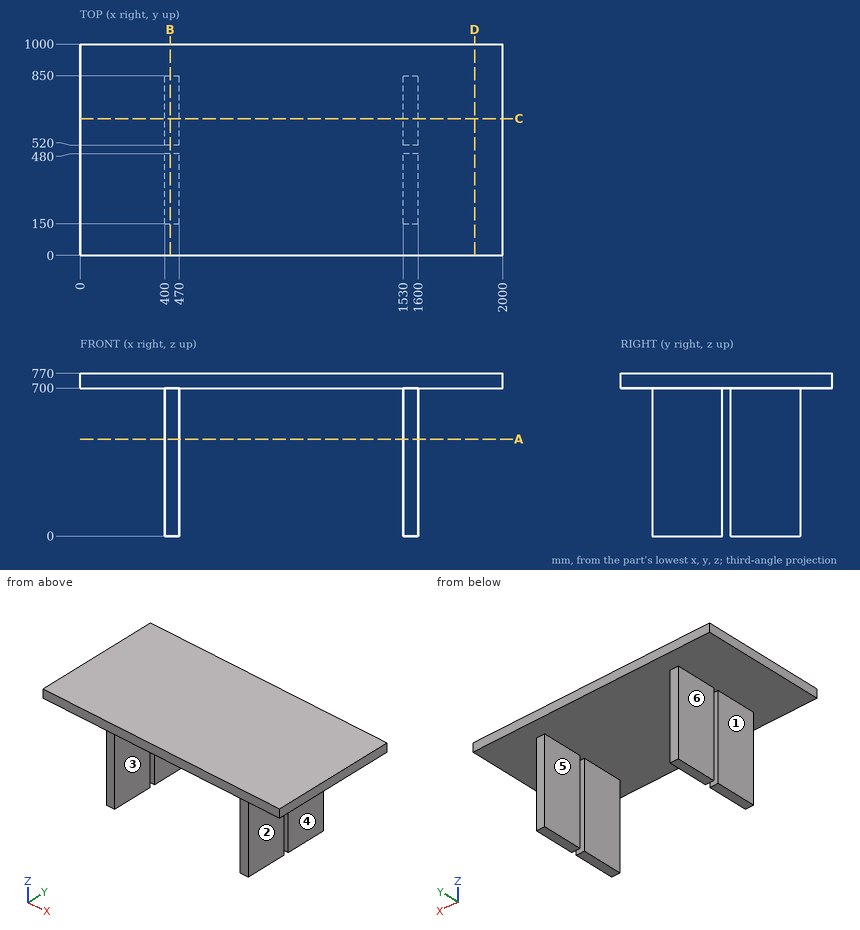
Could you check a few things on this drawing? It's one solid part, dimensions in mm from its lowest x, y, z. A direction names the side the tool comes from. Round coordinates to 2 decimals unless told otherwise and drop trailing zeros. Order: outer loops, then holes, each group sorted by start corner. A loop starts at its lowest first (then second) coordinate and runs counter-clockwise, first axis right, second up.
Q1. Thinking about a two-plate mould opening in X: for the marked faces 1, 2 and 3, which applies, released by +X, released by -X, zero draft, split by the parting line, or undercut?
Geometry says:
face 1: released by -X
face 2: released by +X
face 3: undercut
Q2. Imagine slicing it at C-C, the plane y = 647. List the corners of the cut face in (x, z) for me, then the cut area to 3 significant figures.
Geometry says:
outline: (0, 700) - (400, 700) - (400, 0) - (470, 0) - (470, 700) - (1530, 700) - (1530, 0) - (1600, 0) - (1600, 700) - (2000, 700) - (2000, 770) - (0, 770) - close
area: 238,000 mm2
Q3. Imagine slicing it at A-A, the plane z = 458.5. List the corners of the cut face in (x, y) for me, then the cut area to 3 significant figures.
Geometry says:
outline: (400, 150) - (470, 150) - (470, 480) - (400, 480) - close; (400, 520) - (470, 520) - (470, 850) - (400, 850) - close; (1530, 150) - (1600, 150) - (1600, 480) - (1530, 480) - close; (1530, 520) - (1600, 520) - (1600, 850) - (1530, 850) - close
area: 92,400 mm2
Q4. I'm going to push flat-ended pins straight in: P1, Ø1.5, axis at x = 1175, y = 259, coming from the -Z side; P2, Ø21, axis at x = 1553.5, z = 468, coming from the -Y side; P3, Ø5, axis at y = 422, z = 252, coming from the -X side. Where does each tip first touch, or does it pass through?
Geometry says:
P1: stops at z = 700
P2: stops at y = 150
P3: stops at x = 400
Q5. Imagine slicing it at B-B, the plane x = 426. List the corners of the cut face in (y, z) for me.
Geometry says:
outline: (0, 700) - (150, 700) - (150, 0) - (480, 0) - (480, 700) - (520, 700) - (520, 0) - (850, 0) - (850, 700) - (1000, 700) - (1000, 770) - (0, 770) - close
Q6. Which directions (+Z, -Z, +X, -X, +Y, -Y) give clear straight access to the entire face, cutting with the end or side of a thin tool? Please do the marked faces 4, 5 and 6.
Geometry says:
face 4: -Z, +X, +Y, -Y
face 5: -Z, +Y, -Y
face 6: -Z, -X, +Y, -Y
Q7. Please list where these lines run through material, in increasing order: probe 1 along X at (y, z) = (612.5, 132); probe 2 along Y at (x, z) = (441, 621); probe 3 along Z at (x, y) = (1526.5, 428.5).
Geometry says:
probe 1: x = 400 to 470, 1530 to 1600
probe 2: y = 150 to 480, 520 to 850
probe 3: z = 700 to 770
Q8. Imagine slicing it at D-D, the plane x = 1867. List the corners of the cut face in (y, z) for me, then the cut area to 3 significant figures.
Geometry says:
outline: (0, 700) - (1000, 700) - (1000, 770) - (0, 770) - close
area: 70,000 mm2
